Geometry check sheet. Reference: the model listing, model coordinates, mm. A direction names the side the tool comes from. Round coordinates to 2 decimals unless told otherwise and drop trailing zeros. Order: outer loops, then holes, each group sorted by start corner. A loop starts at its lowest first (then second) coordinate and runs counter-clockwise, first axis right, second up. Notation, with made-up numbers: (45.5, 51.25) -> (58.5, 51.25) arc R21 ccw to (58.5, 62.25) -> close; hole circle Ø8 at (48, -39.5). An arc over 180 degrees is marked (long way). Answer as a JSON object with one key per item and string values. Group by question number.
from build123d import *
from build123d import SkipClean  # not in build123d's __all__

# Parameters (mm, degrees)
F0_R      = 45
F1_DEPTH  = 38.1
F2_R      = 13.9074924411
F3_DEPTH  = 92.41422
F7_R      = 20.32
F8_DEPTH  = 19.05
F9_R      = 20.32
F10_DEPTH = 16.96493
F11_R     = 20.32
F12_DEPTH = 17.20109
F13_R     = 20.32
F14_DEPTH = 19.05
F16_DEPTH = 17.78
F17_W     = 88.86107839
F17_H     = 39.3804269531
F18_DEPTH = 25.4
F19_R     = 22.6323588882
F23_DEPTH = 6.92853
F24_W     = 6.92853
F24_H     = 2.8661746596
F25_DEPTH = 25.4


with BuildPart() as f1:
    # F0 (on Right) → F1 (new body)
    with BuildSketch(Plane.YZ):
        Circle(F0_R)
    extrude(amount=-F1_DEPTH)

    # F2 (on face) → F3 (join)
    with BuildSketch(Plane.YZ):
        Circle(F2_R)
    extrude(amount=F3_DEPTH)

    # F7 (on Right) → F8 (join)
    with BuildSketch(Plane.YZ):
        Circle(F7_R)
    extrude(amount=F8_DEPTH)

    # F9 (on offset) → F10 (join)
    with BuildSketch(Plane.YZ.offset(25.4)):
        Circle(F9_R)
    extrude(amount=F10_DEPTH)

    # F11 (on offset) → F12 (join)
    with BuildSketch(Plane.YZ.offset(45.72)):
        Circle(F11_R)
    extrude(amount=F12_DEPTH)

    # F13 (on offset) → F14 (join)
    with BuildSketch(Plane.YZ.offset(66.04)):
        Circle(F13_R)
    extrude(amount=F14_DEPTH)

    # F15 (on face) → F16 (join)
    with BuildSketch(Plane.YZ.offset(85.09)):
        Polygon((13.7920507069, 14.6662479487), (-5.8053179483, 19.2773902568), (-19.5973686552, 4.6111423081), (-13.7920507069, -14.6662479487), (5.8053179483, -19.2773902568), (19.5973686552, -4.6111423081), align=None)
    extrude(amount=F16_DEPTH)

    # F17 (on face) → F18 (cut)
    with BuildSketch(Plane(origin=(-38.1, 0, 0), x_dir=(0, -1, 0), z_dir=(-1, 0, 0))):
        with Locations((0.0670028883, 27.2318741928)):
            Rectangle(F17_W, F17_H)
        with Locations((0.0670028883, -27.2318741928)):
            Rectangle(F17_W, F17_H)
    extrude(amount=-F18_DEPTH, mode=Mode.SUBTRACT)

    # F19
    f19_edges = [f1.edges().sort_by_distance(p)[0] for p in [
        (-12.7, 0, 7.541661),
        (-12.7, 0, -7.541661),
    ]]
    fillet(f19_edges, radius=F19_R)

    # F20 (on face) → F21 (revolve, cut)
    with BuildSketch(Plane(origin=(-38.1, 0, 0), x_dir=(0, -1, 0), z_dir=(-1, 0, 0))):
        with BuildLine():
            Line((0, -7.5416607163), (0, 0))
            Line((0, 0), (0, 7.5416607163))
            Line((0, 7.5416607163), (-25.8131183102, 7.5416607163))
            ThreePointArc((-25.8131183102, 7.5416607163), (-26.8922614009, 0), (-25.8131183102, -7.5416607163))
            Line((-25.8131183102, -7.5416607163), (0, -7.5416607163))
        make_face()
        with BuildLine():
            Line((-25.8131183102, 7.5416607163), (0, 7.5416607163))
            Line((0, 7.5416607163), (0, 26.8922614009))
            ThreePointArc((0, 26.8922614009), (-16.1304279527, 21.5175049045), (-25.8131183102, 7.5416607163))
        make_face()
        with BuildLine():
            Line((0, -26.8922614009), (0, -7.5416607163))
            Line((0, -7.5416607163), (-25.8131183102, -7.5416607163))
            ThreePointArc((-25.8131183102, -7.5416607163), (-16.1304279527, -21.5175049045), (0, -26.8922614009))
        make_face()
    revolve(axis=Axis((-38.1, 0, 10.4196144343), (0, 0, -1)), mode=Mode.SUBTRACT)

    # F22 (on face) → F23 (join)
    with BuildSketch(Plane(origin=(-38.1, 0, 0), x_dir=(0, -1, 0), z_dir=(-1, 0, 0))):
        with BuildLine():
            Line((-25.8131183102, 7.5416607163), (-44.3635363068, 7.5416607163))
            ThreePointArc((-44.3635363068, 7.5416607163), (-45, 0), (-44.3635363068, -7.5416607163))
            Line((-44.3635363068, -7.5416607163), (-25.8131183102, -7.5416607163))
            ThreePointArc((-25.8131183102, -7.5416607163), (-26.8922614009, 0), (-25.8131183102, 7.5416607163))
        make_face()
        with BuildLine():
            ThreePointArc((25.8131183102, 7.5416607163), (26.8922614009, 0), (25.8131183102, -7.5416607163))
            Line((25.8131183102, -7.5416607163), (44.3635363068, -7.5416607163))
            ThreePointArc((44.3635363068, -7.5416607163), (45, 0), (44.3635363068, 7.5416607163))
            Line((44.3635363068, 7.5416607163), (25.8131183102, 7.5416607163))
        make_face()
    with SkipClean():  # cleaning this boolean's faces spoils the solid; the shape is the same uncleaned
        extrude(amount=F23_DEPTH)

    # F24 (on face) → F25 (cut)
    with BuildSketch(Plane(origin=(0, 0, -7.5416607163), x_dir=(1, 0, 0), z_dir=(0, 0, -1))):
        Polygon((-45.02853, 43.6333455145), (-38.1, 44.3635363068), (-38.1, 47.2297109663), (-45.02853, 47.2297109663), (-45.02853, 44.3635363068), align=None)
        Polygon((-45.02853, -44.3635363068), (-38.1, -44.3635363068), (-45.02853, -43.6333455145), align=None)
        with Locations((-41.564265, -45.7966236366)):
            Rectangle(F24_W, F24_H)
    extrude(amount=-F25_DEPTH, mode=Mode.SUBTRACT)


solid = f1.part
Item 1: Mould release check, pull along Z, two halves, no side actions. Record for faces 6 (the flat face through (93.86, -4.13, -16.94)), 7 (the cylindrical face through (-41.516, -26.892, 0.107)), 8 (the cylindrical face through (-41.516, 26.892, -0.107)), 9 (the flat face through (19.05, -4.8, -13.3)): pulls with the +Z half, pulls with the -Z half, needs draft (parallel to the pull), parting line crosses it, or undercut.
Item 2: Set-up check for faces 1 (the cylindrical face through (22.18, -1.81, 13.79)), 2 (the flat face through (0, 9, -19)), 3 (the flat face through (93.856, -16.735, -4.893)), 4 (the flat face through (93.86, 12.6, -12.05)), 5 (the flat face through (93.856, 16.735, 4.893)): record each of +Z, -Z, +X, -X, +Y, -Y from which the full face is reachable in a straight line by a thin tool's end or side.
Item 3: Sectioned sample at C-C, the plane x = 58. Enter the section's corners in (y, z).
Item 4: Sectioned sample at A-A, the plane x = -31. Enter the section's corners in (y, z).
Item 5: Sectioned sample at D-D, the plane y = 22.5. Enter the section's corners in (x, z) (3 decimals), then the cut area to 3 significant figures.
Item 6: Depth check by flat-ended pin: pin 1 Ø8 at (y, z) = (8, 20) entering from +X; pin 2 Ø12 at (x, z) = (35, 6) entering from -Y; pin 3 Ø0.7 at (y, z) = (45, 2.5) entering from -X; pin 4 Ø7.5 at (y, z) = (0.5, -35) entering from -X. Enter the tip coordinate at first touch or a pass-through.
Item 7: Sectioned sample at B-B, the plane y = 38. Enter the section's corners in (x, z), then the cut area to 3 significant figures.
Item 8: Thickness scan on L1, parallel to X at y = -35, z = -2; L2, parallel to X at y = -26.5, z = 31.5; L3, parallel to X at y = 4.5, z = 16.5. Record the ranges inside material, lowest first.
Result:
{
 "1": {"face 6": "pulls with the -Z half", "face 7": "undercut", "face 8": "undercut", "face 9": "needs draft"},
 "2": {"face 1": "none", "face 2": "+X", "face 3": "-Z, +X, -Y", "face 4": "-Z, +X, +Y", "face 5": "+Z, +X, +Y"},
 "3": {"outline": "circle Ø40.64 at (0, 0)"},
 "4": {"outline": "(-44.29, -7.96) -> (-24.69, -7.96) arc R25.94 cw to (-24.69, 7.96) -> (-44.29, 7.96) arc R45 ccw to start; (24.69, -7.96) -> (44.29, -7.96) arc R45 ccw to (44.29, 7.96) -> (24.69, 7.96) arc R25.94 cw to start"},
 "5": {"outline": "(-26.655, -9.271) arc R22.632 cw to (-12.7, -30.174) -> (-12.7, -38.971) -> (0, -38.971) -> (0, 38.971) -> (-12.7, 38.971) -> (-12.7, 30.174) arc R22.632 cw to (-26.655, 9.271) arc R14.729 cw to start", "area": "1,370 mm2"},
 "6": {"pin 1": "stops at x = 102.87", "pin 2": "stops at y = -20.32", "pin 3": "stops at x = -38.1", "pin 4": "stops at x = -12.7"},
 "7": {"outline": "(-45.03, -7.54) -> (-35.33, -7.54) arc R22.63 cw to (-13.53, -24.1) -> (0, -24.1) -> (0, 24.1) -> (-13.53, 24.1) arc R22.63 cw to (-35.33, 7.54) -> (-45.03, 7.54) -> close", "area": "1,320 mm2"},
 "8": {"L1": "x = -45.03 to 0", "L2": "x = -12.7 to 0", "L3": "x = -17.3 to 19.05, 25.4 to 42.36, 45.72 to 62.92, 66.04 to 102.87"}
}
